```python
from build123d import *

# Parameters (mm, degrees)
SKETCH_1_R             = 12
SKETCH_1_R_2           = 1.515
EXTRUDE_1_DEPTH        = 3
SKETCH_2_R             = 5
EXTRUDE_2_DEPTH        = 23
SKETCH_3_OUTSIDE_W     = 34.552
SKETCH_3_OUTSIDE_H     = 34.552
SKETCH_3_OUTSIDE_R     = 4
CUT_EXTRUDE_1_DEPTH    = 10.1
CHAMFER_1_SIZE         = 0.5
FILLET_1_R             = 0.3
HOLE_WIZARD_M3_1_D     = 2.5
HOLE_WIZARD_M3_1_DEPTH = 9.5
HOLE_WIZARD_M3_1_TIP   = 0.751075774


with BuildPart() as part:
    # 草图1 → 凸台-拉伸1 (new body)
    with BuildSketch(Plane.XY):
        Circle(SKETCH_1_R)
        with Locations((0, 9)):
            Circle(SKETCH_1_R_2, mode=Mode.SUBTRACT)
        with Locations((7.794228634, 4.5)):
            Circle(SKETCH_1_R_2, mode=Mode.SUBTRACT)
        with Locations((7.794228634, -4.5)):
            Circle(SKETCH_1_R_2, mode=Mode.SUBTRACT)
        with Locations((0, -9)):
            Circle(SKETCH_1_R_2, mode=Mode.SUBTRACT)
        with Locations((-7.794228634, -4.5)):
            Circle(SKETCH_1_R_2, mode=Mode.SUBTRACT)
        with Locations((-7.794228634, 4.5)):
            Circle(SKETCH_1_R_2, mode=Mode.SUBTRACT)
    extrude(amount=EXTRUDE_1_DEPTH)

    # 草图2 → 凸台-拉伸2 (add)
    with BuildSketch(Plane.XY.offset(3)):
        Circle(SKETCH_2_R)
    extrude(amount=EXTRUDE_2_DEPTH)

    # 草图3 outside → 切除-拉伸1 (cut)
    with BuildSketch(Plane.XY.offset(26)):
        Rectangle(SKETCH_3_OUTSIDE_W, SKETCH_3_OUTSIDE_H)
        Circle(SKETCH_3_OUTSIDE_R, mode=Mode.SUBTRACT)
    extrude(amount=-CUT_EXTRUDE_1_DEPTH, mode=Mode.SUBTRACT)

    # 倒角1
    chamfer_1_edges = [part.edges().sort_by_distance(p)[0] for p in [
        (-4, 0, 26),
        (-5, 0, 15.9),
    ]]
    chamfer(chamfer_1_edges, length=CHAMFER_1_SIZE)

    # 圆角1
    fillet_1_edges = [part.edges().sort_by_distance(p)[0] for p in [
        (-12, 0, 0),
        (-12, 0, 3),
    ]]
    fillet(fillet_1_edges, radius=FILLET_1_R)

    # M3 螺纹孔1
    with Locations(Plane.XY.offset(26)):
        with Locations((0, 0)):
            Hole(HOLE_WIZARD_M3_1_D / 2, depth=HOLE_WIZARD_M3_1_DEPTH)
            with Locations((0, 0, -(HOLE_WIZARD_M3_1_DEPTH + HOLE_WIZARD_M3_1_TIP / 2))):  # 118° drill point
                Cone(0, HOLE_WIZARD_M3_1_D / 2, HOLE_WIZARD_M3_1_TIP, mode=Mode.SUBTRACT)


solid = part.part
```
Work out the finished part from the listing and answer in its coordinate system (mm). A direction names the side the tool comes from. Give positions to 0.01 mm unless a question says otherwise; leave off trailing zeros. Order: outer loops, then holes, each group sorted by start corner. A loop starts at its lowest first (then second) coordinate and runs counter-clockwise, first axis right, second up. Notation, with made-up numbers: (30, 82.5) - (55, 82.5) arc R14 cw to (55, 107.5) - close; hole circle Ø5 at (19.25, 50). An arc over 180 degrees is marked (long way). One line per item, written item: value. Start each with the question number.
1. Each of these flat-tipped pins is pushed along its axis until it touches: pin 1 Ø10 at (y, z) = (-4, 8.5) entering from +X; pin 2 Ø2.5 at (x, y) = (0, -9) entering from +Z; pin 3 Ø1.5 at (x, z) = (-2, 18.5) entering from -Y; pin 4 Ø4 at (x, y) = (7.79, -4.5) entering from +Z. Where does it stop, or does it pass through?
2. For a pull along X with two mould halves and no side action, classify faces 1 (the face through (6.678, 5.524, 1.479)), 2 (the face through (0, 0, 0)), 3 (the face through (-0.05, -0.21, 15.88)), 4 (the face through (-0.867, -3.905, 20.767)) as released by +X, released by -X, zero draft, split by the parting line, or undercut.
3. Consider line 1 (Y direction, x = 0, z = 1.4) (3 decimals); line 2 (Z direction, x = 5.5, y = -9.75); line 3 (X direction, y = 0, z = 10). Determine where each line is inside the solid, lowest interval first.
4. Section B-B, the plane z = 12 is taken. Write down the section's boundary in (x, y), then the cut area to 3 significant figures.
5. Which of the six approach directions +Z, -Z, +X, -X, +Y, -Y give full straight-line access (tool end or side, diameter ignored) to faces 5 (the face through (5, -2, 3)), 6 (the face through (-11.99, 0.53, 1.48))?
6. Section A-A, the plane z = 22.5 is taken. Write down the section's boundary in (x, y), then the cut area to 3 significant figures.
Filled sheet:
1. pin 1: x = 5
1. pin 2: through
1. pin 3: y = -3.8
1. pin 4: z = 3
2. face 1: undercut
2. face 2: zero draft
2. face 3: undercut
2. face 4: split by the parting line
3. line 1: -12 to -10.515, -7.485 to 7.485, 10.515 to 12
3. line 2: 0 to 3
3. line 3: -5 to 5
4. outline: circle Ø10 at (0, 0)
4. area: 78.5 mm²
5. face 5: +Z
5. face 6: +Z, -Z
6. outline: circle Ø8 at (0, 0); hole circle Ø2.5 at (0, 0)
6. area: 45.4 mm²
